Geometry check sheet. Reference: the model listing, model coordinates, mm. Give positions to 0.01 mm unless a question says otherwise; leave off trailing zeros. Write each loop counter-clockwise with the first axis right and the second up, starting at its lowest first coordinate (ties: lowest second). Pieces come first, ordered by that corner, then holes. Notation, with made-up numbers: M -28.75,-23 L 25.25,-23 A9 ccw 25.25,-11 Z; hole C 2,-34 d3. An arc over 180 degrees is marked long. Use one line per item in the form item = value. Start each with the question number.
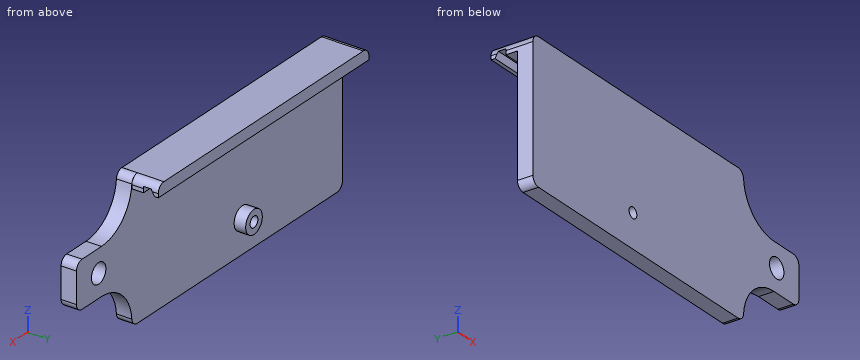
```python
from build123d import *

# Parameters (mm, degrees)
BOSS_EXTRUDE1_DEPTH     = 4
BOSS_EXTRUDE2_DEPTH     = 76
FILLET1_R               = 2
SKETCH3_R               = 3
BOSS_EXTRUDE3_DEPTH     = 3
CUT_EXTRUDE1_DEPTH      = 103.757687
CUT_EXTRUDE1_DEPTH_BACK = 103.757687
SKETCH4_R               = 2.6
SKETCH4_R_2             = 1.4


with BuildPart() as part:
    # Sketch1 → Boss-Extrude1 (new body)
    with BuildSketch(Plane(origin=(0, 0, 0), x_dir=(1, 0, 0), z_dir=(0, 1, 0))):
        with BuildLine():
            Line((2, 0), (74.038519, 0))
            ThreePointArc((74.038519, 0), (75.397251, -0.532401), (76.032593, -1.846154))
            ThreePointArc((76.032593, -1.846154), (79.526972, -9.071793), (87, -12))
            Line((87, -12), (94, -12))
            ThreePointArc((94, -12), (95.414214, -12.585786), (96, -14))
            Line((96, -14), (96, -22))
            ThreePointArc((96, -22), (95.414214, -23.414214), (94, -24))
            Line((94, -24), (87, -24))
            ThreePointArc((87, -24), (79.526972, -26.928207), (76.032593, -34.153846))
            ThreePointArc((76.032593, -34.153846), (75.397251, -35.467599), (74.038519, -36))
            Line((74.038519, -36), (2, -36))
            ThreePointArc((2, -36), (0.585786, -35.414214), (0, -34))
            Line((0, -34), (0, -2))
            ThreePointArc((0, -2), (0.585786, -0.585786), (2, 0))
        make_face()
    extrude(amount=BOSS_EXTRUDE1_DEPTH)

    # Sketch2 → Boss-Extrude2 (add)
    with BuildSketch(Plane.ZY):
        Polygon((36, 4), (36, 10.866025), (33, 10.866025), (33, 9.866025), (34.5, 9), (34.5, 7), (33, 7), (33, 4), align=None)
    extrude(amount=-BOSS_EXTRUDE2_DEPTH)

    # Fillet1
    # the kernel refuses this fillet: 2 mm, written as the material it takes off along each edge
    with BuildSketch(Plane(origin=(0, -1, 36), x_dir=(0, 0, -1), z_dir=(0, 1, 0))) as fillet1_piece_1:
        with BuildLine():
            CenterArc((FILLET1_R, -FILLET1_R), FILLET1_R, 90, 90)
            Line((0, -FILLET1_R), (0, 0))
            Line((0, 0), (FILLET1_R, 0))
        make_face()
    extrude(amount=16.866025, mode=Mode.SUBTRACT)
    with BuildSketch(Plane(origin=(76, -1, 36), x_dir=(-1, 0, 0), z_dir=(0, 1, 0))) as fillet1_piece_2_section:
        with BuildLine():
            CenterArc((FILLET1_R, -FILLET1_R), FILLET1_R, 90, 90)
            Line((0, -FILLET1_R), (0, 0))
            Line((0, 0), (FILLET1_R, 0))
        make_face()
    fillet1_piece_2 = extrude(amount=16.866025, mode=Mode.PRIVATE)
    fillet1_piece_2 = fillet1_piece_2 - Plane(origin=(74.038519, 2, 34), x_dir=(0.9970370305242855, 0, 0.07692307692308645), z_dir=(0, -1, 0)) * Cylinder(2, 42, mode=Mode.PRIVATE)
    add(fillet1_piece_2, mode=Mode.SUBTRACT)
    with BuildSketch(Plane(origin=(76, 4, 36), x_dir=(-1, 0, 0), z_dir=(0, 1, 0))) as fillet1_piece_3:
        with BuildLine():
            CenterArc((FILLET1_R, -FILLET1_R), FILLET1_R, 90, 90)
            Line((0, -FILLET1_R), (0, 0))
            Line((0, 0), (FILLET1_R, 0))
        make_face()
    extrude(amount=11.866025, mode=Mode.SUBTRACT)

    # Sketch3 → Boss-Extrude3 (add)
    with BuildSketch(Plane(origin=(0, 4, 0), x_dir=(1, 0, 0), z_dir=(0, 1, 0))):
        with Locations(Location((36.1, -8.7, 0), (0, 0, 270))):
            Circle(SKETCH3_R)
    extrude(amount=BOSS_EXTRUDE3_DEPTH)

    # Sketch4 → Cut-Extrude1 (cut, two sides: drawn at the far end of the back side and taken through both)
    with BuildSketch(Plane(origin=(0, 4, 0), x_dir=(1, 0, 0), z_dir=(0, 1, 0)).offset(-CUT_EXTRUDE1_DEPTH_BACK)):
        with Locations(Location((88, -18, 0), (0, 0, 270))):
            Circle(SKETCH4_R)
        with Locations(Location((36.1, -8.7, 0), (0, 0, 270))):
            Circle(SKETCH4_R_2)
    extrude(amount=CUT_EXTRUDE1_DEPTH + CUT_EXTRUDE1_DEPTH_BACK, mode=Mode.SUBTRACT)


solid = part.part
```
(1) Depth check by flat-ended pin: pin 1 (0.9 mm diameter, centred on x = 53.5, y = 5.5, fed in from -Z); pin 2 (4 mm diameter, centred on y = 4.5, z = 29, fed in from +X); pin 3 (6 mm diameter, centred on x = 88, z = 18, fed in from +Y). Enter the tip coordinate at first touch or a pass-through.
(2) Sectioned sample at A-A, the plane y = 6. Record the boundary of the cut face in (x, z).
(3) Sectioned sample at C-C, the plane z = 18. Record the boundary of the cut face in (x, y), plus the area to 3 significant figures.
(4) Sectioned sample at B-B, the plane x = 36.1. Record the boundary of the cut face in (y, z).
(5) Sectioned sample at D-D, the plane x = 18.5. Record the boundary of the cut face in (y, z).
(6) Thickness scan on probe 1 along X at (y, z) = (1.5, 18); probe 2 along Z at (x, y) = (88, 1.7); probe 3 along X at (y, z) = (4.5, 8.7). Record the ranges inside material, lowest first. Write a range as [from, to].
Numbers:
q1.pin_1 = 33
q1.pin_2 = 79.38
q1.pin_3 = 4
q2.outline = M 0,33 L 76,33 L 76,34 A2 ccw 74,36 L 2,36 A2 ccw 0,34 Z; C 36.1,8.7 d6; hole C 36.1,8.7 d2.8
q3.outline = M 0,0 L 85.4,0 L 85.4,4 L 0,4 Z; M 90.6,0 L 96,0 L 96,4 L 90.6,4 Z
q3.area = 363 mm2
q4.outline = M 0,0 L 4,0 L 4,5.7 L 7,5.7 L 7,7.3 L 0,7.3 Z; M 0,10.1 L 7,10.1 L 7,11.7 L 4,11.7 L 4,33 L 7,33 L 7,34.5 L 9,34.5 L 9.87,33 L 10.87,33 L 10.87,36 L 0,36 Z
q5.outline = M 0,0 L 4,0 L 4,33 L 7,33 L 7,34.5 L 9,34.5 L 9.87,33 L 10.87,33 L 10.87,36 L 0,36 Z
q6.probe_1 = [0, 85.4], [90.6, 96]
q6.probe_2 = [12, 15.4], [20.6, 24]
q6.probe_3 = [33.1, 34.7], [37.5, 39.1]
